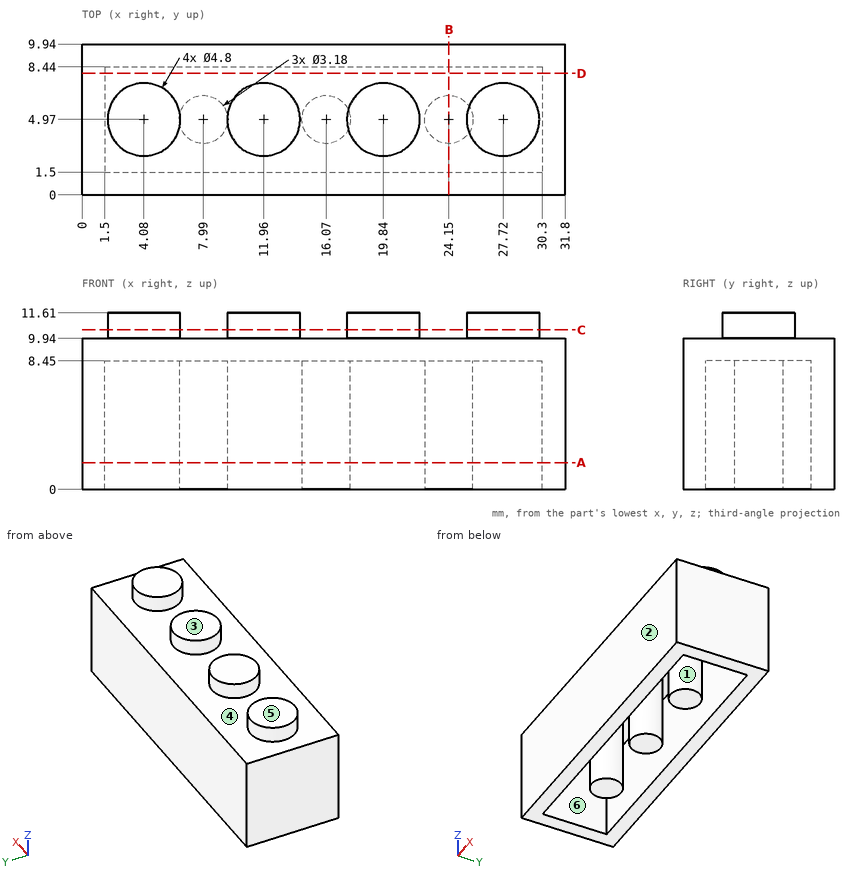
Job drawing, mm, ordinate dimensions from the low corner. One solid piece. A direction names the side the tool comes from. Give positions to 0.01 mm unless a question says otherwise; leave off trailing zeros. Write each loop counter-clockwise with the first axis right and the second up, starting at its lowest first coordinate (ties: lowest second). Pieces come first, ordered by that corner, then holes. Notation, with made-up numbers: (-33, 63) -> (-3, 63) arc R18 ccw to (-3, 81) -> close; hole circle Ø8 at (49.25, -31). An arc over 180 degrees is marked (long way). Return JSON: item names as keys, results as strings.
Item 1: Band-saw the part on D-D (y = 8). List the corners of the cut face in (x, z).
Answer below:
{"outline": "(0, 0) -> (1.5, 0) -> (1.5, 8.45) -> (30.3, 8.45) -> (30.3, 0) -> (31.8, 0) -> (31.8, 9.94) -> (0, 9.94) -> close"}
Item 2: Tool access for the marked faces 4, 5 and 6: list every direction of +Z, -Z, +X, -X, +Y, -Y with a clear straight run to the whole face (end or side of a thin tool).
Answer below:
{"face 4": "+Z", "face 5": "+Z, +X, -X, +Y, -Y", "face 6": "-Z"}
Item 3: Drill centre lines: probe 1 along Y at (x, z) = (8, 5.75); probe 2 along X at (y, z) = (2, 6.25); probe 3 along X at (y, z) = (5, 7.75). Where is each one in solid material? Low to high.
Answer below:
{"probe 1": "y = 0 to 1.5, 3.38 to 6.56, 8.44 to 9.94", "probe 2": "x = 0 to 1.5, 30.3 to 31.8", "probe 3": "x = 0 to 1.5, 6.4 to 9.58, 14.48 to 17.66, 22.56 to 25.74, 30.3 to 31.8"}
Item 4: Band-saw the part on B-B (x = 24.15). List the corners of the cut face in (y, z), then the cut area to 3 significant figures.
Answer below:
{"outline": "(0, 0) -> (1.5, 0) -> (1.5, 8.45) -> (3.38, 8.45) -> (3.38, 0) -> (6.56, 0) -> (6.56, 8.45) -> (8.44, 8.45) -> (8.44, 0) -> (9.94, 0) -> (9.94, 9.94) -> (0, 9.94) -> close", "area": "67.0 mm2"}
Item 5: Band-saw the part on A-A (z = 1.75). List the corners of the cut face in (x, y).
Answer below:
{"outline": "(0, 0) -> (31.8, 0) -> (31.8, 9.94) -> (0, 9.94) -> close; circle Ø3.18 at (7.99, 4.97); circle Ø3.18 at (16.07, 4.97); circle Ø3.18 at (24.15, 4.97); hole (1.5, 1.5) -> (30.3, 1.5) -> (30.3, 8.44) -> (1.5, 8.44) -> close"}
Item 6: Two-plate mould, pull along Y, no slides. Class the marked faces 1, 2 and 3: +Y half, -Y half, draft (parallel to the pull), parting line (faces both ways), or undercut.
Answer below:
{"face 1": "undercut", "face 2": "-Y half", "face 3": "draft"}
Item 7: Band-saw the part on C-C (z = 10.5). List the corners of the cut face in (x, y).
Answer below:
{"outline": "circle Ø4.8 at (4.08, 4.97); circle Ø4.8 at (11.96, 4.97); circle Ø4.8 at (19.84, 4.97); circle Ø4.8 at (27.72, 4.97)"}
